```python
from build123d import *

# Parameters (mm, degrees)
F0_W      = 20
F0_H      = 20
F1_DEPTH  = 20
F2_W      = 20
F2_H      = 20
F2_R      = 2.6
F3_DEPTH  = 1
F4_R      = 2.6
F5_DEPTH  = 1
F6_R      = 2.6
F7_DEPTH  = 1
F9_R      = 2.6
F10_DEPTH = 1
F11_R     = 2.6
F12_DEPTH = 1
F14_R     = 2.6
F15_DEPTH = 1
F16_R     = 0.5


with BuildPart() as f1:
    # F0 (on Front) → F1 (new body)
    with BuildSketch(Plane.XZ):
        with Locations((10, 10)):
            Rectangle(F0_W, F0_H)
    extrude(amount=F1_DEPTH)

    # F2 (on face) → F3 (join)
    with BuildSketch(Plane.XZ.offset(20)):
        with Locations((10, 10)):
            Rectangle(F2_W, F2_H)
        with Locations((10, 10)):
            Circle(F2_R, mode=Mode.SUBTRACT)
    extrude(amount=F3_DEPTH)

    # F4 (on face) → F5 (cut)
    with BuildSketch(Plane(origin=(0, 0, 0), x_dir=(0, -1, 0), z_dir=(-1, 0, 0))):
        with Locations((6.5558182063, 13.2910121384)):
            Circle(F4_R)
        with Locations((14.9031878165, 6.3120640028)):
            Circle(F4_R)
    extrude(amount=-F5_DEPTH, mode=Mode.SUBTRACT)

    # F6 (on face) → F7 (cut)
    with BuildSketch(Plane.XY.offset(20)):
        with Locations((5.2196445889, -5.4806268184)):
            Circle(F6_R)
        with Locations((15.0386817887, -5.2093841219)):
            Circle(F6_R)
        with Locations((5.2196445889, -15.5193731816)):
            Circle(F6_R)
        with Locations((15.0386817887, -15.7906158781)):
            Circle(F6_R)
    extrude(amount=-F7_DEPTH, mode=Mode.SUBTRACT)

    # F9 (on face) → F10 (cut)
    with BuildSketch(Plane(origin=(0, 0, 0), x_dir=(1, 0, 0), z_dir=(0, 0, -1))):
        with Locations((4.7041235123, 4.8818840855)):
            Circle(F9_R)
        with Locations((10.0668108718, 10.4472179903)):
            Circle(F9_R)
        with Locations((15.2967504263, 15.8747877835)):
            Circle(F9_R)
    extrude(amount=-F10_DEPTH, mode=Mode.SUBTRACT)

    # F11 (on face) → F12 (cut)
    with BuildSketch(Plane(origin=(0, 0, 0), x_dir=(-1, 0, 0), z_dir=(0, 1, 0))):
        with Locations((-15.4185416177, 3.2414922025)):
            Circle(F11_R)
        with Locations((-15.7072935253, 10.5565581471)):
            Circle(F11_R)
        with Locations((-15.5147919431, 16.7166125029)):
            Circle(F11_R)
        with Locations((-4.4852080569, 16.7166125029)):
            Circle(F11_R)
        with Locations((-4.2927064747, 10.5565581471)):
            Circle(F11_R)
        with Locations((-4.5814583823, 3.2414922025)):
            Circle(F11_R)
    extrude(amount=-F12_DEPTH, mode=Mode.SUBTRACT)

    # F14 (on face) → F15 (cut)
    with BuildSketch(Plane.YZ.offset(20)):
        with Locations((-16.1984862848, 4.3908170937)):
            Circle(F14_R)
        with Locations((-10.3718864697, 9.9916504576)):
            Circle(F14_R)
        with Locations((-16.2744057865, 15.5611082293)):
            Circle(F14_R)
        with Locations((-4.7255942135, 15.5611082293)):
            Circle(F14_R)
        with Locations((-4.8015137152, 4.3908170937)):
            Circle(F14_R)
    extrude(amount=-F15_DEPTH, mode=Mode.SUBTRACT)

    # F16
    f16_edges = [f1.edges().sort_by_distance(p)[0] for p in [
        (10, -21, 0),
        (20, -21, 10),
        (20, -10.5, 0),
        (20, 0, 10),
        (10, 0, 0),
        (20, -10.5, 20),
        (7.4, -21, 10),
        (10, -21, 20),
        (0, -10.5, 20),
        (10, 0, 20),
        (0, 0, 10),
        (0, -21, 10),
        (0, -10.5, 0),
    ]]
    fillet(f16_edges, radius=F16_R)


solid = f1.part
```
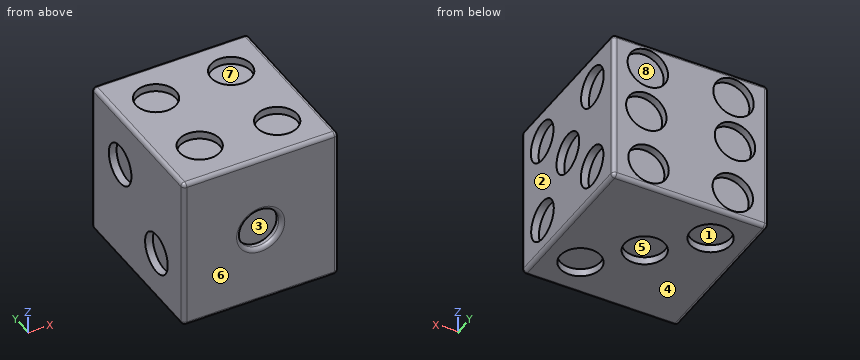
Part model, mm, in its own coordinate system. Face numbers are marked on the shaded views. A direction names the side the tool comes from. Coordinates: 2 decimals unless noted, no trailing zeros. Write each loop counter-clockwise with the first axis right and the second up, starting at its lowest first coordinate (ties: lowest second). Pieces come first, ordered by that corner, then holes.
Item 1: Pin check, flat tips, straight feed: pin 1 (4 mm diameter, centred on y = -17, z = 3.5, fed in from +X); pin 2 (1.6 mm diameter, centred on x = 16, z = 18, fed in from +Y); pin 3 (2.5 mm diameter, centred on y = -11, z = 9, fed in from +X); pin 4 (3 mm diameter, centred on x = 5.22, y = -5.48, fed in from -Z). Stop position of each tip, or through.
Item 2: Mould opens along Z. For the marked faces 1, 2 and 3 say: released by +Z, released by -Z, zero draft, split by the parting line, or undercut.
Item 3: Probe line 1 (Z direction, x = 10, y = -20.1); line 2 (Y direction, x = 14, z = 4.5); line 3 (X direction, y = -16.25, z = 16). List the from-to ranges inside material, lowest first.
Item 4: Slice it at C-C (x = 10). Write the cut outline in (y, z).
Item 5: Which spindle directions (+Z, -Z, +X, -X, +Y, -Y) get a long thin tool onto all of the face, cutting with end or side? Do the marked faces 4, 5, 6, 7 and 8. Say none if no direction does.
Results found:
1. pin 1: stops at x = 20
1. pin 2: stops at y = -1
1. pin 3: stops at x = 19
1. pin 4: stops at z = 1
2. face 1: released by -Z
2. face 2: zero draft
2. face 3: undercut
3. line 1: z = 0 to 7.4, 12.6 to 20
3. line 2: y = -21 to -1
3. line 3: x = 0 to 19
4. outline: (-21, 0.5) arc R0.5 ccw to (-20.5, 0) - (-13.05, 0) - (-13.05, 1) - (-7.85, 1) - (-7.85, 0) - (-0.5, 0) arc R0.5 ccw to (0, 0.5) - (0, 19.5) arc R0.5 ccw to (-0.5, 20) - (-20.5, 20) arc R0.5 ccw to (-21, 19.5) - (-21, 13.1) arc R0.5 ccw to (-20.5, 12.6) - (-20, 12.6) - (-20, 7.4) - (-20.5, 7.4) arc R0.5 ccw to (-21, 6.9) - close
5. face 4: -Z, +X, -X, +Y, -Y
5. face 5: -Z
5. face 6: +Z, -Z, +X, -X, -Y
5. face 7: +Z
5. face 8: +Y
